For this review, use the dimensioned drawing (mm, ordinates from the lowest corner) and the shaded views. A direction names the side the tool comes from. Give positions to 0.01 mm unless a question says otherwise; leave off trailing zeros. Write each loop counter-clockwise with the first axis right and the second up, starting at its lowest first coordinate (ties: lowest second). Pieces come first, ordered by that corner, then holes. Notation, with made-up numbers: M -4,16 L 20,16 A24 ccw 20,42 Z; hole C -34,71.25 d7. An arc over 180 degrees is marked long. Answer in a Markdown table with one row per item.
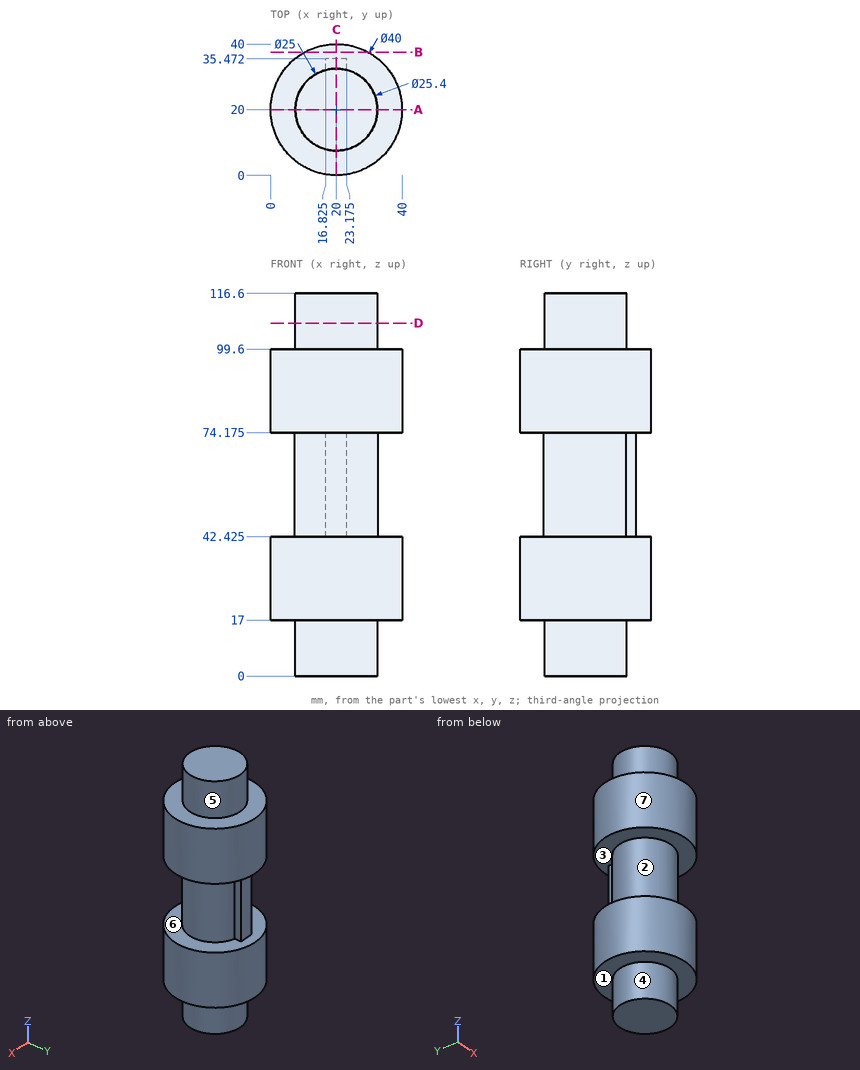
1) Add section A-A (y = 20). Write out the cut boundary in (x, z) (1 decimal).
Geometry says:
| item | result |
|---|---|
| outline | M 0,17 L 7.5,17 L 7.5,0 L 32.5,0 L 32.5,17 L 40,17 L 40,42.4 L 32.7,42.4 L 32.7,74.2 L 40,74.2 L 40,99.6 L 32.5,99.6 L 32.5,116.6 L 7.5,116.6 L 7.5,99.6 L 0,99.6 L 0,74.2 L 7.3,74.2 L 7.3,42.4 L 0,42.4 Z |
2) Insertion check: P1, Ø2.5, axis at y = 34.5, z = 63, coming from the -X side (3 decimals); P2, Ø3, axis at y = 17, z = 72, coming from the -X side; P3, Ø2, axis at x = 35, y = 16, coming from the -Z side. Each pin has a flat end and moves straight along its axis. Give the tip position at first contact, or say it passes through.
Geometry says:
| item | result |
|---|---|
| P1 | x = 16.825 |
| P2 | x = 7.39 |
| P3 | z = 17 |
3) Add section B-B (y = 37.5). Write out the cut boundary in (x, z) (1 decimal).
Geometry says:
| item | result |
|---|---|
| outline | M 10.3,17 L 29.7,17 L 29.7,42.4 L 10.3,42.4 Z; M 10.3,74.2 L 29.7,74.2 L 29.7,99.6 L 10.3,99.6 Z |
4) For the marked faces 5, 6 and 7, list the 3-axis set-ups (+Z, -Z, +X, -X, +Y, -Y) from which the entire face can be reached by the end or side of a thin tool; tool diameter is ignored.
Geometry says:
| item | result |
|---|---|
| face 5 | +Z |
| face 6 | none |
| face 7 | +Z, -Z |
5) To check wall thickness, follow probe 1 along Z at (x, y) = (32, 25) (1 decimal); probe 2 along Y at (x, z) = (19.5, 31); probe 3 along X at (y, z) = (33, 34). State the ranges of each line that lie inside material, in increasing order. Write a range as [from, to].
Geometry says:
| item | result |
|---|---|
| probe 1 | [17, 42.4], [74.2, 99.6] |
| probe 2 | [0.01, 39.99] |
| probe 3 | [4.8, 35.2] |
6) Add section C-C (x = 20). Write out the cut boundary in (y, z) (1 decimal).
Geometry says:
| item | result |
|---|---|
| outline | M 0,17 L 7.5,17 L 7.5,0 L 32.5,0 L 32.5,17 L 40,17 L 40,42.4 L 35.5,42.4 L 35.5,74.2 L 40,74.2 L 40,99.6 L 32.5,99.6 L 32.5,116.6 L 7.5,116.6 L 7.5,99.6 L 0,99.6 L 0,74.2 L 7.3,74.2 L 7.3,42.4 L 0,42.4 Z |
7) The part is to be moulded in two halves that separate along Z. For the marked faces 1, 2, 3 and 4, say which applies: released by +Z, released by -Z, zero draft, split by the parting line, or undercut.
Geometry says:
| item | result |
|---|---|
| face 1 | released by -Z |
| face 2 | undercut |
| face 3 | undercut |
| face 4 | zero draft |
8) Add section D-D (z = 107.5). Write out the cut boundary in (x, y), and give its area (3 significant figures).
Geometry says:
| item | result |
|---|---|
| outline | C 20,20 d25 |
| area | 491 mm^2 |
